```python
from build123d import *

# Parameters (mm, degrees)
F1_DEPTH       = 300
F3_D           = 4.5
F3_CBORE_D     = 8.25
F3_CBORE_DEPTH = 4


with BuildPart() as f1:
    # F0 (on Front) → F1 (new body)
    with BuildSketch(Plane.XZ):
        with BuildLine():
            Line((-6.5, -6.75), (6.5, -6.75))
            Line((6.5, -6.75), (7.5, -5.75))
            Line((7.5, -5.75), (7.5, -2.75))
            Line((7.5, -2.75), (7.2, -2.75))
            Line((7.2, -2.75), (7.2, -2.45))
            Line((7.2, -2.45), (7.2, -0.05))
            Line((7.2, -0.05), (7.2, 0.25))
            Line((7.2, 0.25), (7.5, 0.25))
            Line((7.5, 0.25), (7.5, 2.75))
            ThreePointArc((7.5, 2.75), (7.3535533906, 3.1035533906), (7, 3.25))
            Line((7, 3.25), (5.5, 3.25))
            ThreePointArc((5.5, 3.25), (5.1464466094, 3.3964466094), (5, 3.75))
            Line((5, 3.75), (5, 4.25))
            ThreePointArc((5, 4.25), (5.1464466094, 4.6035533906), (5.5, 4.75))
            Line((5.5, 4.75), (7, 4.75))
            ThreePointArc((7, 4.75), (7.3535533906, 4.8964466094), (7.5, 5.25))
            Line((7.5, 5.25), (7.5, 5.75))
            Line((7.5, 5.75), (6.5, 6.75))
            Line((6.5, 6.75), (-6.5, 6.75))
            Line((-6.5, 6.75), (-7.5, 5.75))
            Line((-7.5, 5.75), (-7.5, 5.25))
            ThreePointArc((-7.5, 5.25), (-7.3535533906, 4.8964466094), (-7, 4.75))
            Line((-7, 4.75), (-5.5, 4.75))
            ThreePointArc((-5.5, 4.75), (-5.1464466094, 4.6035533906), (-5, 4.25))
            Line((-5, 4.25), (-5, 3.75))
            ThreePointArc((-5, 3.75), (-5.1464466094, 3.3964466094), (-5.5, 3.25))
            Line((-5.5, 3.25), (-7, 3.25))
            ThreePointArc((-7, 3.25), (-7.3535533906, 3.1035533906), (-7.5, 2.75))
            Line((-7.5, 2.75), (-7.5, 0.25))
            Line((-7.5, 0.25), (-7.2, 0.25))
            Line((-7.2, 0.25), (-7.2, -0.05))
            Line((-7.2, -0.05), (-7.2, -2.45))
            Line((-7.2, -2.45), (-7.2, -2.75))
            Line((-7.2, -2.75), (-7.5, -2.75))
            Line((-7.5, -2.75), (-7.5, -5.75))
            Line((-7.5, -5.75), (-6.5, -6.75))
        make_face()
        Polygon((-7.2, 0.25), (-7.5, 0.25), (-7.2, -0.05), align=None)
        Polygon((-7.2, -2.45), (-7.5, -2.75), (-7.2, -2.75), align=None)
        Polygon((7.2, -2.75), (7.5, -2.75), (7.2, -2.45), align=None)
        Polygon((7.2, -0.05), (7.5, 0.25), (7.2, 0.25), align=None)
    extrude(amount=-F1_DEPTH)

    # F3 (through all)
    with Locations(Plane.XY.offset(6.75)):
        with Locations((0, 20), (0, 80), (0, 140), (0, 200), (0, 260)):
            CounterBoreHole(F3_D / 2, F3_CBORE_D / 2, F3_CBORE_DEPTH)


solid = f1.part
```
Part model, mm, in its own coordinate system. A direction names the side the tool comes from. Round coordinates to 2 decimals unless told otherwise and drop trailing zeros. Use CSV: the item, a comma, the result in double quotes. Start each with the question number.
1) Pull direction X, two halves, no side cores. Call faces 3 (the cylindrical face through (-1, 256, 5)), 4 (the flat face through (0, 148, 6.75)): +X half, -X half, draft (parallel to the pull), parting line (faces both ways), or undercut.
2) Cut at A-A, the plane x = 0. Give the number of separate pieces and of enclosed holes in the cut face, plus the area to 3 significant figures.
3) Which spindle directions (+Z, -Z, +X, -X, +Y, -Y) get a long thin tool onto all of the face, cutting with end or side? Do faces 1 (the flat face through (0, 148, -6.75)), 2 (the flat face through (2, 138, 2.75)). Say none if no direction does.
4) Drop flat-ended pins along their axis: P1, Ø6.5, axis at x = 0, y = 80, coming from the +Z side; P2, Ø1.2, axis at y = 210, z = -1.5, coming from the +X side. Give the stop position or say it passes through.
5) Wall check: L1, parallel to Y at x = 0, z = 5.15 (3 decimals); L2, parallel to Z at x = 6.5, y = 257. Give the ranges that are in metal, low to high. Write a range as [from, to].
Determined:
1,face 3,"undercut"
1,face 4,"draft"
2,separate pieces,"6"
2,enclosed holes,"0"
2,area,"3,670 mm2"
3,face 1,"-Z, +X, -X, +Y, -Y"
3,face 2,"+Z"
4,P1,"stops at z = 2.75"
4,P2,"stops at x = 7.2"
5,L1,"y = [0, 15.875], [24.125, 75.875], [84.125, 135.875], [144.125, 195.875], [204.125, 255.875], [264.125, 300]"
5,L2,"z = [-6.75, 3.25], [4.75, 6.75]"
